Could you check a few things on this model? Use its own coordinates, in mm. Face numbers are marked on the shaded views. Round coordinates to 2 decimals unless told otherwise and drop trailing zeros. Return JSON: item names as keys, results as strings. Group by question number.
```python
from build123d import *

# Parameters (mm, degrees)
F3_R     = 25
F4_DEPTH = 142.02346
F5_R     = 1675.475624
F5_R_2   = 1433.116866
F6_DEPTH = 100


with BuildPart() as f2:
    # F1 (on Front) → F2 (revolve)
    with BuildSketch(Plane.XZ):
        with BuildLine():
            Line((-326.189038, -696.030591), (-340.047231, -690.29034))
            Line((-340.047231, -690.29034), (-646.193977, -1429.393966))
            ThreePointArc((-646.193977, -1429.393966), (-646.193977, -1467.662309), (-619.134172, -1494.722114))
            Line((-619.134172, -1494.722114), (-613.39392, -1480.863921))
            ThreePointArc((-613.39392, -1480.863921), (-632.335784, -1461.922058), (-632.335784, -1435.134217))
            Line((-632.335784, -1435.134217), (-326.189038, -696.030591))
        make_face()
    revolve(axis=Axis((-300, 0, -724.264069), (-0.382683, 0, -0.92388)))

    # F3 (on Front) → F4 (cut, symmetric)
    with BuildSketch(Plane.XZ):
        with Locations((-600, -1448.528137)):
            Circle(F3_R)
    extrude(amount=F4_DEPTH, both=True, mode=Mode.SUBTRACT)

    # F5 (on Front) → F6 (cut)
    with BuildSketch(Plane.XZ):
        Circle(F5_R)
        Circle(F5_R_2, mode=Mode.SUBTRACT)
    extrude(amount=F6_DEPTH, mode=Mode.SUBTRACT)


solid = f2.part
```
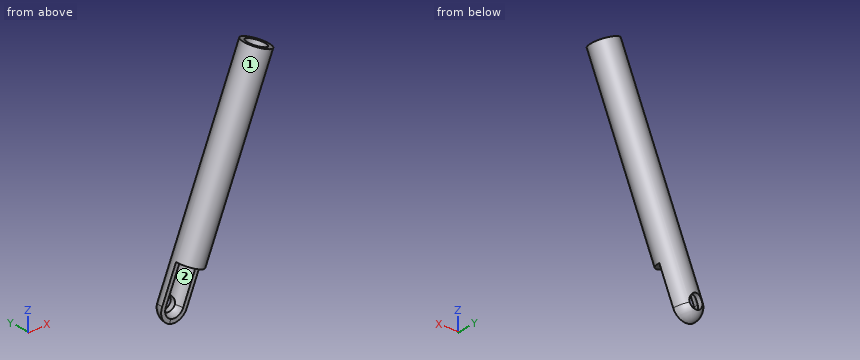
1. I'm going to push flat-ended pins straight in: pin 1 Ø3 at (y, z) = (37.5, -1233) entering from -X; pin 2 Ø3 at (y, z) = (25, -1394) entering from -X; pin 3 Ø1.5 at (y, z) = (-8, -1214.5) entering from +X. Where does each tip first touch, or does it pass through?
2. I need wall thicknesses on probe 1 along Y at (x, z) = (-467.5, -1127.5); probe 2 along Y at (x, z) = (-414.5, -954.5); probe 3 along X at (y, z) = (28, -1404). Which ranges of each line are inside material? Lowest first, please.
3. We'd pull the mould along Y, two halves only. Please class the marked faces 1 and 2: +Y half, -Y half, draft (parallel to the pull), parting line (faces both ways), or undercut.
Geometry results:
{
 "1": {"pin 1": "x = -548.39", "pin 2": "x = -625.38", "pin 3": "x = -449.3"},
 "2": {"probe 1": "-50 to -35, 35 to 50", "probe 2": "-46.77 to -30.21, 30.21 to 46.77", "probe 3": "-626.39 to -604.29, -558.82 to -536.72"},
 "3": {"face 1": "parting line", "face 2": "undercut"}
}
